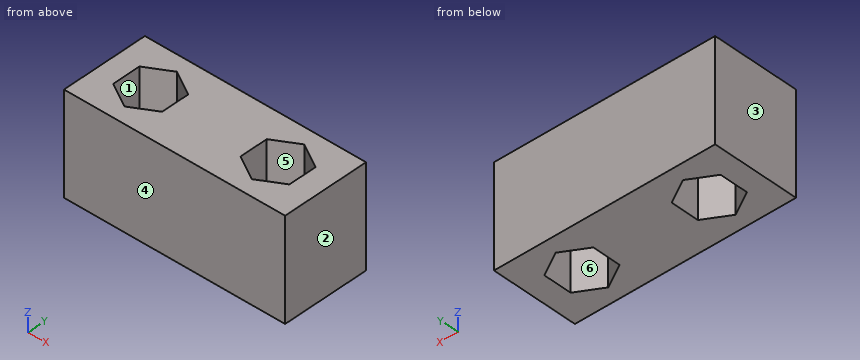
Solid Edge part; units mm, degrees
sketch "Sketch1" plane through (0, 0, 0) normal (0, 0, 1) x (1, 0, 0)
  line L0 (-28.65, 2.1155) -> (-25, 4.2228)
  line L1 (-25, 4.2228) -> (-21.35, 2.1155)
  line L2 (-21.35, 2.1155) -> (-21.35, -2.0992)
  line L3 (-21.35, -2.0992) -> (-25, -4.2065)
  line L4 (-25, -4.2065) -> (-28.65, -2.0992)
  line L5 (-28.65, -2.0992) -> (-28.65, 2.1155)
  line L6 (-50.9022, 6.5) -> (-17.9022, 6.5)
  line L7 (-17.9022, 6.5) -> (-17.9022, -6.5)
  line L8 (-17.9022, -6.5) -> (-50.9022, -6.5)
  line L9 (-50.9022, -6.5) -> (-50.9022, 6.5)
  line L10 (-47.65, 2.1155) -> (-44, 4.2228)
  line L11 (-44, 4.2228) -> (-40.35, 2.1155)
  line L12 (-40.35, 2.1155) -> (-40.35, -2.0992)
  line L13 (-40.35, -2.0992) -> (-44, -4.2065)
  line L14 (-44, -4.2065) -> (-47.65, -2.0992)
  line L15 (-47.65, -2.0992) -> (-47.65, 2.1155)
extrude "Protrusion1" add sketch "Sketch1" along normal mid plane 15
CAD build for the part. Positions are in the model's coordinates, mm. Face numbers are marked on the shaded views. A direction names the side the tool comes from. Coordinates: 2 decimals unless noted, no trailing zeros. Write each loop counter-clockwise with the first axis right and the second up, starting at its lowest first coordinate (ties: lowest second). Pieces come first, ordered by that corner, then holes. Notation, with made-up numbers: (49.25, -30.75) -> (55.25, -30.75) arc R25 cw to (55.25, -8.75) -> close; hole circle Ø7 at (-39.5, -36). An arc over 180 degrees is marked (long way). Return JSON: item names as keys, results as strings. Group by question number.
Q1. Cut at A-A, the plane y = 0.5. Give the cut face in (x, z), then the cut area to 3 significant figures.
Q2. Drill centre lines: line 1 (X direction, y = -1.75, z = -2.75); line 2 (X direction, y = 3.25, z = 0); line 3 (Y direction, x = -43, z = 5.75). Where is each one in solid material? Low to high.
Q3. Pull direction X, two halves, no side cores. Call the marked faces 3, 4, 5 and 6: released by +X, released by -X, zero draft, split by the parting line, or undercut.
Q4. Cut at B-B, the plane x = -43. Give the cut face in (y, z), then the cut area to 3 significant figures.
Q5. Cut at D-D, the plane y = -2.75. Give the cut face in (x, z), then the cut area to 3 significant figures.
Q6. Which spindle directions (+Z, -Z, +X, -X, +Y, -Y) get a long thin tool onto all of the face, cutting with end or side? Do the marked faces 1 and 2. Say none if no direction does.
Q7. Cut at C-C, the plane z = -2.5. Give the cut face in (x, y), then the cut area to 3 significant figures.
Returned:
{
 "1": {"outline": "(-50.9, -7.5) -> (-47.65, -7.5) -> (-47.65, 7.5) -> (-50.9, 7.5) -> close; (-40.35, -7.5) -> (-28.65, -7.5) -> (-28.65, 7.5) -> (-40.35, 7.5) -> close; (-21.35, -7.5) -> (-17.9, -7.5) -> (-17.9, 7.5) -> (-21.35, 7.5) -> close", "area": "276 mm2"},
 "2": {"line 1": "x = -50.9 to -47.65, -40.35 to -28.65, -21.35 to -17.9", "line 2": "x = -50.9 to -45.68, -42.32 to -26.68, -23.32 to -17.9", "line 3": "y = -6.5 to -3.63, 3.65 to 6.5"},
 "3": {"face 3": "released by -X", "face 4": "zero draft", "face 5": "undercut", "face 6": "undercut"},
 "4": {"outline": "(-6.5, -7.5) -> (-3.63, -7.5) -> (-3.63, 7.5) -> (-6.5, 7.5) -> close; (3.65, -7.5) -> (6.5, -7.5) -> (6.5, 7.5) -> (3.65, 7.5) -> close", "area": "85.9 mm2"},
 "5": {"outline": "(-50.9, -7.5) -> (-46.52, -7.5) -> (-46.52, 7.5) -> (-50.9, 7.5) -> close; (-41.48, -7.5) -> (-27.52, -7.5) -> (-27.52, 7.5) -> (-41.48, 7.5) -> close; (-22.48, -7.5) -> (-17.9, -7.5) -> (-17.9, 7.5) -> (-22.48, 7.5) -> close", "area": "344 mm2"},
 "6": {"face 1": "+Z, -Z", "face 2": "+Z, -Z, +X, +Y, -Y"},
 "7": {"outline": "(-50.9, -6.5) -> (-17.9, -6.5) -> (-17.9, 6.5) -> (-50.9, 6.5) -> close; hole (-47.65, -2.1) -> (-44, -4.21) -> (-40.35, -2.1) -> (-40.35, 2.12) -> (-44, 4.22) -> (-47.65, 2.12) -> close; hole (-28.65, -2.1) -> (-25, -4.21) -> (-21.35, -2.1) -> (-21.35, 2.12) -> (-25, 4.22) -> (-28.65, 2.12) -> close", "area": "337 mm2"}
}
